Check sheet for the modelled part. Datum: model origin and axes. Units: mm. A direction names the side the tool comes from. Give positions to 0.01 mm unless a question says otherwise; leave off trailing zeros. Order: outer loops, then holes, each group sorted by start corner. A loop starts at its lowest first (then second) coordinate and runs counter-clockwise, first axis right, second up. Notation, with made-up numbers: (79.25, 89.25) -> (124.25, 89.25) arc R18 cw to (124.25, 112.25) -> close; hole circle Ø5 at (0, 33). An arc over 180 degrees is marked (long way). Answer in a Markdown table with one row per item. Add a question column.
(1) Release check for a two-part mould opening along Z. For faces 1 (the face through (2, 2, 6)), 2 (the face through (0, -2, 9)), 3 (the face through (0, 0, 0)) record: released by +Z, released by -Z, zero draft, split by the parting line, or undercut.
(2) Cross-section at A-A (y = -1). Record the cut outline in (x, z), then the cut area to 3 significant figures.
(3) Thickness scan on L1, parallel to Z at x = -1.05, y = -3; L2, parallel to Y at x = -1.1, z = 3.5. Record the ranges inside material, lowest first. Write a range as [from, to].
(4) Cross-section at B-B (x = -1.5). Record the cut outline in (y, z).
(5) Set-up check for faces 4 (the face through (0, 1, 6)), 5 (the face through (0, 5, 6)): record each of +Z, -Z, +X, -X, +Y, -Y from which the full face is reachable in a straight line by a thin tool's end or side.
(6) Go/stop test with flat-tipped pins: pin 1 (4 mm diameter, centred on y = 0.5, z = 3.5, fed in from -X); pin 2 (2 mm diameter, centred on x = -1, z = 6.5, fed in from -Y); pin 3 (4 mm diameter, centred on y = -3.5, z = 6, fed in from -X). Record where each tip stops, or that it passes through.
(7) Cross-section at C-C (z = 3.5). Record the cut outline in (x, y), then the cut area to 3 significant figures.
```python
from build123d import *

# Parameters (mm, degrees)
F0_W     = 4
F0_H     = 4
F0_H_2   = 6
F1_DEPTH = 12
F2_DEPTH = 9
F3_DEPTH = 3


with BuildPart() as f1:
    # F0 (on Top) → F1 (new body)
    with BuildSketch(Plane.XY):
        with Locations((0, 3)):
            Rectangle(F0_W, F0_H)
        with Locations((0, -2)):
            Rectangle(F0_W, F0_H_2)
    extrude(amount=F1_DEPTH)

    # F0 (on Top) → F2 (cut)
    with BuildSketch(Plane.XY):
        with Locations((0, -2)):
            Rectangle(F0_W, F0_H_2)
    extrude(amount=F2_DEPTH, mode=Mode.SUBTRACT)

    # F0 (on Top) → F3 (join)
    with BuildSketch(Plane.XY):
        with Locations((0, -2)):
            Rectangle(F0_W, F0_H_2)
    extrude(amount=F3_DEPTH)


solid = f1.part
```
Answer below:
| question | item | result |
|---|---|---|
| 1 | face 1 | zero draft |
| 1 | face 2 | undercut |
| 1 | face 3 | released by -Z |
| 2 | outline | (-2, 0) -> (2, 0) -> (2, 3) -> (-2, 3) -> close; (-2, 9) -> (2, 9) -> (2, 12) -> (-2, 12) -> close |
| 2 | area | 24.0 mm² |
| 3 | L1 | z = [0, 3], [9, 12] |
| 3 | L2 | y = [1, 5] |
| 4 | outline | (-5, 0) -> (5, 0) -> (5, 12) -> (-5, 12) -> (-5, 9) -> (1, 9) -> (1, 3) -> (-5, 3) -> close |
| 5 | face 4 | +X, -X, -Y |
| 5 | face 5 | +Z, -Z, +X, -X, +Y |
| 6 | pin 1 | stops at x = -2 |
| 6 | pin 2 | stops at y = 1 |
| 6 | pin 3 | passes through |
| 7 | outline | (-2, 1) -> (2, 1) -> (2, 5) -> (-2, 5) -> close |
| 7 | area | 16.0 mm² |
